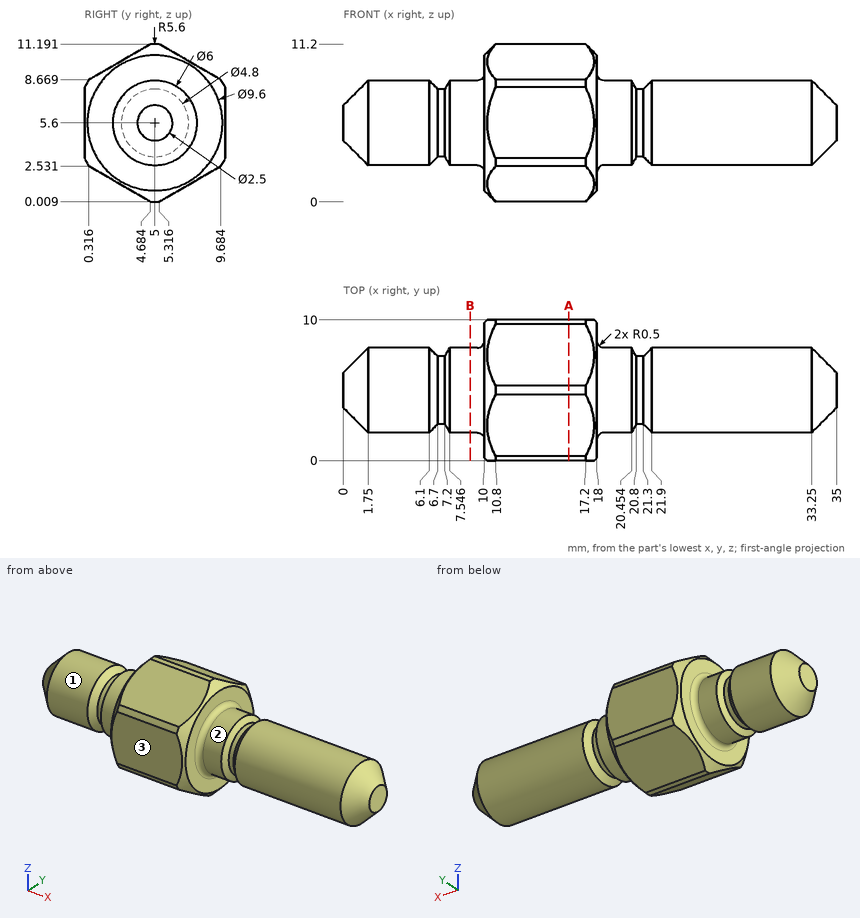
Job drawing, mm, ordinate dimensions from the low corner. One solid piece. A direction names the side the tool comes from. Round coordinates to 2 decimals unless told otherwise and drop trailing zeros. Loops run counter-clockwise (first coordinate to the right, second up) from the corner with the lowest first, then second, coordinate; pieces in that order, holes last. Notation, with made-up numbers: (-7.75, 80.5) -> (0.25, 80.5) arc R15 cw to (0.25, 103.5) -> close; hole circle Ø11 at (25.25, 11). An arc over 180 degrees is marked (long way). Use a Markdown table: item, result.
1) Drop flat-ended pins along their axis: pin 1 Ø5 at (y, z) = (8.5, 4) entering from +X; pin 2 Ø2 at (x, z) = (28, 7.5) entering from +Y; pin 3 Ø1 at (x, z) = (20.5, 7.5) entering from +Y. Give the stop position or say it passes through.
The answers:
| item | result |
|---|---|
| pin 1 | stops at x = 34.9 |
| pin 2 | stops at y = 7.86 |
| pin 3 | stops at y = 7.65 |
2) Cut at A-A, the plane x = 16. List the corners of the cut face in (y, z).
The answers:
| item | result |
|---|---|
| outline | (0, 3.08) arc R5.6 ccw to (0.32, 2.53) -> (4.68, 0.01) arc R5.6 ccw to (5.32, 0.01) -> (9.68, 2.53) arc R5.6 ccw to (10, 3.08) -> (10, 8.12) arc R5.6 ccw to (9.68, 8.67) -> (5.32, 11.19) arc R5.6 ccw to (4.68, 11.19) -> (0.32, 8.67) arc R5.6 ccw to (0, 8.12) -> close |
3) Tool access for the marked faces 1, 2 and 3: list every direction of +Z, -Z, +X, -X, +Y, -Y with a clear straight run to the whole face (end or side of a thin tool).
The answers:
| item | result |
|---|---|
| face 1 | -X |
| face 2 | +X |
| face 3 | +Z, -Z, +X, -X, -Y |
4) Cut at B-B, the plane x = 9. List the corners of the cut face in (y, z).
The answers:
| item | result |
|---|---|
| outline | circle Ø6 at (5, 5.6) |
5) Probe line 1 (X direction, y = 6.75, z = 3.75) (1 decimal); line 2 (Z direction, x = 30.5, y = 5); line 3 (X direction, y = 7.5, z = 2.5). List the from-to ranges inside material, lowest first. Write a range as [from, to].
The answers:
| item | result |
|---|---|
| line 1 | x = [1.3, 6.6], [7.3, 20.7], [21.4, 33.7] |
| line 2 | z = [2.6, 8.6] |
| line 3 | x = [10, 18] |
